Could you check a few things on this model? Use its own coordinates, in mm. A direction names the side the tool comes from. Give positions to 0.01 mm unless a question says otherwise; leave off trailing zeros. Order: outer loops, then holes, each group sorted by start corner. A loop starts at its lowest first (then second) coordinate and runs counter-clockwise, first axis right, second up.
(1) Imagine slicing it at A-A, the plane z = 63. Write out the boundary of the cut face in (x, y), then the cut area to 3 significant figures.
(2) If I drill on probe 1 along X at (y, z) = (24, 9.5); probe 2 along Y at (x, z) = (-21.5, 63); probe 3 along Z at (x, y) = (42.5, 79), over which ranges is the centre line in solid material (lowest first)?
(3) If we mould it in two halves opening along X, with no side actions, what happens to faces 4 (the flat face through (45.944, 88.514, 2.958)), 5 (the flat face through (22, 78, 6)), 6 (the flat face through (22, 77, 0))? For each: released by +X, released by -X, zero draft, split by the parting line, or undercut.
(4) Will these pins go through, and if not, where does the flat tip stop? pin 1 (23 mm diameter, centred on y = 16.5, z = 25.5, fed in from +X); pin 2 (6 mm diameter, centred on x = 11.5, y = 5, fed in from +Z); pin 3 (5.5 mm diameter, centred on x = -35, y = 81.21, fed in from -Z); pin 4 (3 mm diameter, centred on x = 14, z = 85.5, fed in from +Y).
(5) Imagine slicing it at C-C, the plane x = 0. Write out the boundary of the cut face in (y, z).
(6) On a 3-axis mill with a long thin cutter (end or side, diameter ignored), from which of +Z, -Z, +X, -X, +Y, -Y can I reach the whole of each face in a straight line? I mean faces 1 (the cylindrical face through (34.83, -3, 16.75)), 2 (the flat face through (-48.42, 19.22, 20.3)), 3 (the flat face through (46.9, 11, 14)). Say none if no direction works.
(7) Imagine slicing it at B-B, the plane x = -35. Write out the boundary of the cut face in (y, z), then the cut area to 3 significant figures.
(8) Imagine slicing it at D-D, the plane y = 72.5. Write out the boundary of the cut face in (x, z).
from build123d import *

# Parameters (mm, degrees)
SKETCH1_W           = 100
SKETCH1_H           = 98.5
SKETCH1_R           = 36.5
SKETCH1_R_2         = 3.4
BOSS_EXTRUDE1_DEPTH = 6
SKETCH2_W           = 100
SKETCH2_H           = 6
BOSS_EXTRUDE2_DEPTH = 92.5
CHAMFER1_SIZE       = 8
CUT_EXTRUDE1_DEPTH  = 145.078103819
BOSS_EXTRUDE3_START = -0.1
BOSS_EXTRUDE3_DEPTH = 3
BOSS_EXTRUDE4_START = -0.1
BOSS_EXTRUDE4_DEPTH = 3
FILLET1_R           = 2


with BuildPart() as part:
    # Sketch1 → Boss-Extrude1 (new body)
    with BuildSketch(Plane.XY):
        with Locations((0, 43.207953426)):
            Rectangle(SKETCH1_W, SKETCH1_H)
        with Locations((0, 46.207953426)):
            Circle(SKETCH1_R, mode=Mode.SUBTRACT)
        with Locations((-35, 81.207953426)):
            Circle(SKETCH1_R_2, mode=Mode.SUBTRACT)
        with Locations((35, 81.207953426)):
            Circle(SKETCH1_R_2, mode=Mode.SUBTRACT)
        with Locations((35, 11.207953426)):
            Circle(SKETCH1_R_2, mode=Mode.SUBTRACT)
        with Locations((-35, 11.207953426)):
            Circle(SKETCH1_R_2, mode=Mode.SUBTRACT)
    extrude(amount=BOSS_EXTRUDE1_DEPTH)

    # Sketch2 → Boss-Extrude2 (add)
    with BuildSketch(Plane.XY.offset(6)):
        with Locations((0, -3.042046574)):
            Rectangle(SKETCH2_W, SKETCH2_H)
    extrude(amount=BOSS_EXTRUDE2_DEPTH)

    # Chamfer1
    chamfer1_edges = [part.edges().sort_by_distance(p)[0] for p in [
        (-50, -3.042046574, 98.5),
        (50, -3.042046574, 98.5),
        (-50, 92.457953426, 3),
        (50, 92.457953426, 3),
    ]]
    chamfer(chamfer1_edges, length=CHAMFER1_SIZE)

    # Sketch3 → Cut-Extrude1 (cut, through all)
    with BuildSketch(Plane(origin=(0, -0.042046574, 0), x_dir=(1, 0, 0), z_dir=(0, 1, 0))):
        with BuildLine():
            Line((-38.25, -84.25), (-38.25, -20.25))
            ThreePointArc((-38.25, -20.25), (-34.75, -16.75), (-31.25, -20.25))
            Line((-31.25, -20.25), (-31.25, -84.25))
            ThreePointArc((-31.25, -84.25), (-34.75, -87.75), (-38.25, -84.25))
        make_face()
        with BuildLine():
            Line((38.25, -84.25), (38.25, -20.25))
            ThreePointArc((38.25, -20.25), (34.75, -16.75), (31.25, -20.25))
            Line((31.25, -20.25), (31.25, -84.25))
            ThreePointArc((31.25, -84.25), (34.75, -87.75), (38.25, -84.25))
        make_face()
    extrude(amount=-CUT_EXTRUDE1_DEPTH, mode=Mode.SUBTRACT)

    # Sketch4 → Boss-Extrude3 (add)
    with BuildSketch(Plane.ZY.offset(50).offset(BOSS_EXTRUDE3_START)):
        Polygon((6, 37.957953426), (35, -0.042046574), (12.357101974, -0.042046574), (6, 8.287949116), align=None)
    extrude(amount=-BOSS_EXTRUDE3_DEPTH)

    # Sketch5 → Boss-Extrude4 (add)
    with BuildSketch(Plane(origin=(50, 0, 0), x_dir=(0, 0, -1), z_dir=(1, 0, 0)).offset(BOSS_EXTRUDE4_START)):
        Polygon((-6, 8.287949116), (-6, 37.957953426), (-35, -0.042046574), (-12.357101974, -0.042046574), align=None)
    extrude(amount=-BOSS_EXTRUDE4_DEPTH)

    # Fillet1
    fillet1_edges = [part.edges().sort_by_distance(p)[0] for p in [
        (0, -0.042046574, 6),
        (0, -6.042046574, 0),
    ]]
    fillet(fillet1_edges, radius=FILLET1_R)


solid = part.part
Answer block:
1. outline: (-50, -6.04) - (-38.25, -6.04) - (-38.25, -0.04) - (-50, -0.04) - close; (-31.25, -6.04) - (31.25, -6.04) - (31.25, -0.04) - (-31.25, -0.04) - close; (38.25, -6.04) - (50, -6.04) - (50, -0.04) - (38.25, -0.04) - close
1. area: 516 mm2
2. probe 1: x = -49.9 to -46.9, 46.9 to 49.9
2. probe 2: y = -6.04 to -0.04
2. probe 3: z = 0 to 6
3. face 4: released by +X
3. face 5: undercut
3. face 6: zero draft
4. pin 1: stops at x = 49.9
4. pin 2: stops at z = 6
4. pin 3: passes through
4. pin 4: stops at y = -0.04
5. outline: (-6.04, 2) arc R2 ccw to (-4.04, 0) - (9.71, 0) - (9.71, 6) - (1.96, 6) arc R2 cw to (-0.04, 8) - (-0.04, 98.5) - (-6.04, 98.5) - close; (82.71, 0) - (92.46, 0) - (92.46, 6) - (82.71, 6) - close
6. face 1: +Y, -Y
6. face 2: +Z, +X, -X, +Y
6. face 3: +Z, +Y
7. outline: (-6.04, 2) arc R2 ccw to (-4.04, 0) - (7.81, 0) - (7.81, 6) - (1.96, 6) arc R2 cw to (-0.04, 8) - (-0.04, 16.76) - (-6.04, 16.76) - close; (-6.04, 87.74) - (-0.04, 87.74) - (-0.04, 98.5) - (-6.04, 98.5) - close; (14.61, 0) - (35.85, 0) - (35.85, 6) - (14.61, 6) - close; (56.56, 0) - (77.81, 0) - (77.81, 6) - (56.56, 6) - close; (84.61, 0) - (92.46, 0) - (92.46, 6) - (84.61, 6) - close
7. area: 514 mm2
8. outline: (-50, 0) - (-25.32, 0) - (-25.32, 6) - (-50, 6) - close; (25.32, 0) - (50, 0) - (50, 6) - (25.32, 6) - close
